The listing builds one solid part. Answer for the finished solid, in the listing's coordinates (mm). Coordinates: 2 decimals unless noted, no trailing zeros. Loops run counter-clockwise (first coordinate to the right, second up) from the corner with the lowest first, then second, coordinate; pieces in that order, holes last. Notation, with made-up numbers: (32, 12.25) - (81, 12.25) arc R21 ccw to (81, 19.25) - close; hole circle Ø7 at (52.5, -6.5). An arc over 180 degrees is marked (long way). Return JSON: item names as keys, results as strings. Group by question number.
1. Section B-B (y = 3.75) is taken. State how many separate pieces and enclosed holes the cut face has, and give its area (3 significant figures).
2. Find the intervals of material crossed by line 1 along Z through (x, y) = (9.5, 6.5); line 2 along X through (y, z) = (5.75, -430.5); line 3 along Z through (x, y) = (14.75, 6.5), in increasing order.
3. Section A-A (z = -408.5) is taken. Write down the section's boundary in (x, y).
4. This flat-tipped pin is pushed along its axis until it touches: P1, Ø1.8, axis at x = 4.5, z = -15.09, coming from the -Y side. Where does it stop, or does it pass through?
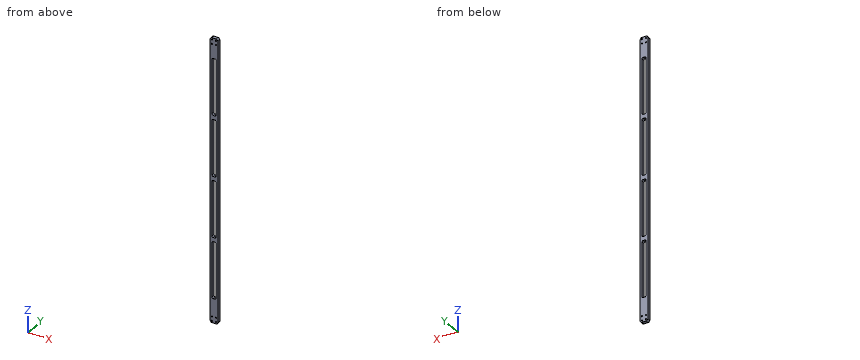
```python
from build123d import *

# Parameters (mm, degrees)
SKETCH_1_R          = 1.5
EXTRUDE_1_DEPTH     = 8
CUT_EXTRUDE_2_DEPTH = 701.303505632


with BuildPart() as part:
    # 草图1 → 凸台-拉伸1 (new body)
    with BuildSketch(Plane(origin=(0, 0, 0), x_dir=(1, 0, 0), z_dir=(0, 1, 0))):
        with BuildLine():
            Line((4.5, 0), (14.5, 0))
            ThreePointArc((14.5, 0), (17.681980515, 1.318019485), (19, 4.5))
            Line((19, 4.5), (19, 695.5))
            ThreePointArc((19, 695.5), (17.681980515, 698.681980515), (14.5, 700))
            Line((14.5, 700), (4.5, 700))
            ThreePointArc((4.5, 700), (1.318019485, 698.681980515), (0, 695.5))
            Line((0, 695.5), (0, 4.5))
            ThreePointArc((0, 4.5), (1.318019485, 1.318019485), (4.5, 0))
        make_face()
        with Locations(Location((4.5, 4.5, 0), (0, 0, 270))):
            Circle(SKETCH_1_R, mode=Mode.SUBTRACT)
        with Locations(Location((14.5, 4.5, 0), (0, 0, 270))):
            Circle(SKETCH_1_R, mode=Mode.SUBTRACT)
        with Locations(Location((4.5, 15.08659859, 0), (0, 0, 270))):
            Circle(SKETCH_1_R, mode=Mode.SUBTRACT)
        with Locations(Location((14.5, 15.08659859, 0), (0, 0, 270))):
            Circle(SKETCH_1_R, mode=Mode.SUBTRACT)
        with Locations(Location((14.5, 684.91340141, 0), (0, 0, 90))):
            Circle(SKETCH_1_R, mode=Mode.SUBTRACT)
        with Locations(Location((4.5, 684.91340141, 0), (0, 0, 90))):
            Circle(SKETCH_1_R, mode=Mode.SUBTRACT)
        with Locations(Location((14.5, 695.5, 0), (0, 0, 90))):
            Circle(SKETCH_1_R, mode=Mode.SUBTRACT)
        with Locations(Location((4.5, 695.5, 0), (0, 0, 90))):
            Circle(SKETCH_1_R, mode=Mode.SUBTRACT)
    extrude(amount=EXTRUDE_1_DEPTH)

    # 草图5 → 切除-拉伸2 (cut, through all)
    with BuildSketch(Plane(origin=(0, 8, 0), x_dir=(1, 0, 0), z_dir=(0, 1, 0))):
        with BuildLine():
            Line((7.5, 50), (11.5, 50))
            ThreePointArc((11.5, 50), (13.621320344, 50.878679656), (14.5, 53))
            Line((14.5, 53), (14.5, 187))
            ThreePointArc((14.5, 187), (13.621320344, 189.121320344), (11.5, 190))
            Line((11.5, 190), (7.5, 190))
            ThreePointArc((7.5, 190), (5.378679656, 189.121320344), (4.5, 187))
            Line((4.5, 187), (4.5, 53))
            ThreePointArc((4.5, 53), (5.378679656, 50.878679656), (7.5, 50))
        make_face()
        with BuildLine():
            Line((14.5, 203), (14.5, 337))
            ThreePointArc((14.5, 337), (13.621320344, 339.121320344), (11.5, 340))
            Line((11.5, 340), (7.5, 340))
            ThreePointArc((7.5, 340), (5.378679656, 339.121320344), (4.5, 337))
            Line((4.5, 337), (4.5, 203))
            ThreePointArc((4.5, 203), (5.378679656, 200.878679656), (7.5, 200))
            Line((7.5, 200), (11.5, 200))
            ThreePointArc((11.5, 200), (13.621320344, 200.878679656), (14.5, 203))
        make_face()
        with BuildLine():
            Line((14.5, 353), (14.5, 487))
            ThreePointArc((14.5, 487), (13.621320344, 489.121320344), (11.5, 490))
            Line((11.5, 490), (7.5, 490))
            ThreePointArc((7.5, 490), (5.378679656, 489.121320344), (4.5, 487))
            Line((4.5, 487), (4.5, 353))
            ThreePointArc((4.5, 353), (5.378679656, 350.878679656), (7.5, 350))
            Line((7.5, 350), (11.5, 350))
            ThreePointArc((11.5, 350), (13.621320344, 350.878679656), (14.5, 353))
        make_face()
        with BuildLine():
            Line((14.5, 503), (14.5, 637))
            ThreePointArc((14.5, 637), (13.621320344, 639.121320344), (11.5, 640))
            Line((11.5, 640), (7.5, 640))
            ThreePointArc((7.5, 640), (5.378679656, 639.121320344), (4.5, 637))
            Line((4.5, 637), (4.5, 503))
            ThreePointArc((4.5, 503), (5.378679656, 500.878679656), (7.5, 500))
            Line((7.5, 500), (11.5, 500))
            ThreePointArc((11.5, 500), (13.621320344, 500.878679656), (14.5, 503))
        make_face()
    extrude(amount=-CUT_EXTRUDE_2_DEPTH, mode=Mode.SUBTRACT)


solid = part.part
```
The answers:
{
 "1": {"separate pieces": "1", "enclosed holes": "12", "area": "7,660 mm2"},
 "2": {"line 1": "z = -700 to -640, -500 to -490, -350 to -340, -200 to -190, -50 to 0", "line 2": "x = 0 to 4.5, 14.5 to 19", "line 3": "z = -699.99 to -696.98, -694.02 to -686.39, -683.43 to -16.57, -13.61 to -5.98, -3.02 to -0.01"},
 "3": {"outline": "(0, 0) - (4.5, 0) - (4.5, 8) - (0, 8) - close; (14.5, 0) - (19, 0) - (19, 8) - (14.5, 8) - close"},
 "4": {"P1": "passes through"}
}
